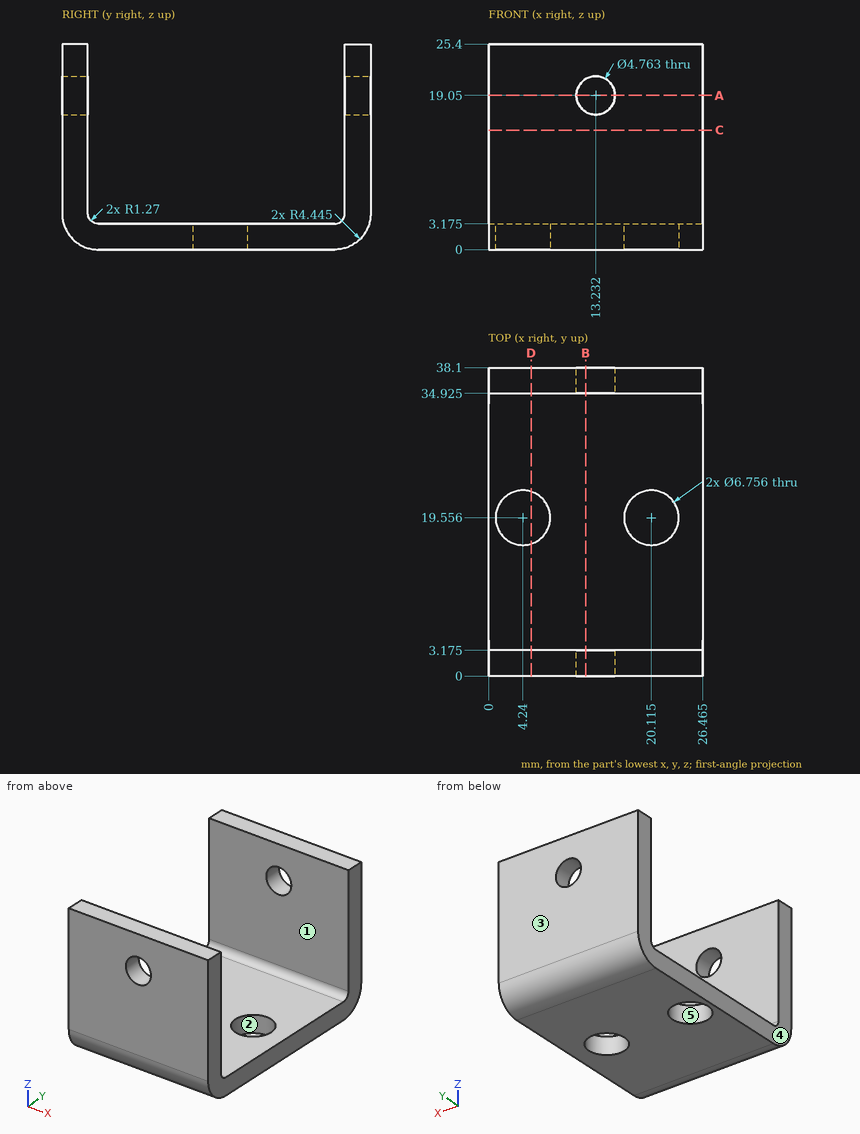
Check sheet for the drawn part. Datum: minimum x, y, z corner. Units: mm. A direction names the side the tool comes from. Give positions to 0.01 mm unless a question says otherwise; leave off trailing zeros. Write each loop counter-clockwise with the first axis right and the second up, starting at its lowest first coordinate (ties: lowest second). Pieces come first, ordered by that corner, then holes. Notation, with made-up numbers: (-13.5, -27.75) -> (33.5, -27.75) arc R26 ccw to (33.5, -7.75) -> close; hole circle Ø9 at (26, 85). An arc over 180 degrees is marked (long way). Use one line per item in the form item = value. Start each with the question number.
1. Section check D-D (x = 5.25). Record the cut outline in (y, z) (1 decimal).
2. Go/stop test with flat-tipped pins: P1, Ø5, axis at x = 9, y = 6, coming from the +Z side (1 decimal); P2, Ø4, axis at x = 5.5, y = 8, coming from the +Z side (3 decimals). Record where each tip stops, or that it passes through.
3. Access from +Z, -Z, +X, -X, +Y, -Y to the whole of each face (thin tool, end or side, straight path). Record for the marked faces 1 and 2.
4. Section check B-B (x = 12). Record the cut outline in (y, z) (1 decimal).
5. Mould release check, pull along Y, two halves, no side actions. Record for the marked faces 3, 4 and 5: pulls with the +Y half, pulls with the -Y half, needs draft (parallel to the pull), parting line crosses it, or undercut.
6. Thickness scan on line 1 along X through (y, z) = (37.3, 19.05) (1 decimal); line 2 along Y through (x, z) = (6.5, 6.5) (1 decimal); line 3 along Z through (x, y) = (12.5, 30.5) (1 decimal). Record the ranges inside material, lowest first. Write a range as from..to.
7. Section check C-C (z = 14.75). Record the cut outline in (x, y) (1 decimal), and give its area (3 significant figures).
8. Section check A-A (z = 19.05). Record the cut outline in (x, y) (1 decimal).
Conclusion:
q1.outline = (0, 4.4) arc R4.4 ccw to (4.4, 0) -> (16.3, 0) -> (16.3, 3.2) -> (4.4, 3.2) arc R1.3 cw to (3.2, 4.4) -> (3.2, 25.4) -> (0, 25.4) -> close; (22.8, 0) -> (33.7, 0) arc R4.4 ccw to (38.1, 4.4) -> (38.1, 25.4) -> (34.9, 25.4) -> (34.9, 4.4) arc R1.3 cw to (33.7, 3.2) -> (22.8, 3.2) -> close
q2.P1 = 3.6
q2.P2 = 3.175
q3.face_1 = +Z, +X, -X
q3.face_2 = +Z, -Z
q4.outline = (0, 4.4) arc R4.4 ccw to (4.4, 0) -> (33.7, 0) arc R4.4 ccw to (38.1, 4.4) -> (38.1, 17) -> (34.9, 17) -> (34.9, 4.4) arc R1.3 cw to (33.7, 3.2) -> (4.4, 3.2) arc R1.3 cw to (3.2, 4.4) -> (3.2, 17) -> (0, 17) -> close; (0, 21.1) -> (3.2, 21.1) -> (3.2, 25.4) -> (0, 25.4) -> close; (34.9, 21.1) -> (38.1, 21.1) -> (38.1, 25.4) -> (34.9, 25.4) -> close
q5.face_3 = pulls with the +Y half
q5.face_4 = needs draft
q5.face_5 = undercut
q6.line_1 = 0..10.9, 15.6..26.5
q6.line_2 = 0..3.2, 34.9..38.1
q6.line_3 = 0..3.2
q7.outline = (0, 0) -> (26.5, 0) -> (26.5, 3.2) -> (0, 3.2) -> close; (0, 34.9) -> (26.5, 34.9) -> (26.5, 38.1) -> (0, 38.1) -> close
q7.area = 168 mm²
q8.outline = (0, 0) -> (10.9, 0) -> (10.9, 3.2) -> (0, 3.2) -> close; (0, 34.9) -> (10.9, 34.9) -> (10.9, 38.1) -> (0, 38.1) -> close; (15.6, 0) -> (26.5, 0) -> (26.5, 3.2) -> (15.6, 3.2) -> close; (15.6, 34.9) -> (26.5, 34.9) -> (26.5, 38.1) -> (15.6, 38.1) -> close
